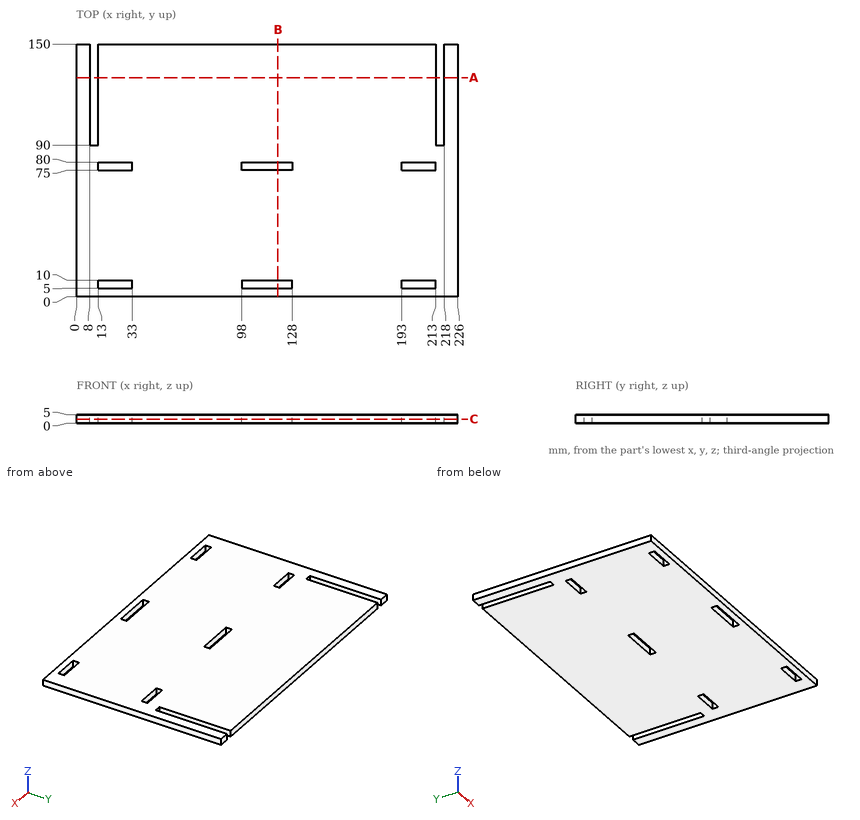
Study the drawing (mm; zero at the part's minimum x, y, z) and answer. Round coordinates to 2 decimals unless told otherwise and drop trailing zeros. Write each loop counter-clockwise with the first axis right and the second up, starting at its lowest first coordinate (ties: lowest second). Pieces come first, ordered by that corner, then holes.
Q1. Find section A-A on y = 130. Determine the outline of the cut face in (x, z), and give its area (3 significant figures).
Values:
outline: (0, 0) - (8, 0) - (8, 5) - (0, 5) - close; (13, 0) - (213, 0) - (213, 5) - (13, 5) - close; (218, 0) - (226, 0) - (226, 5) - (218, 5) - close
area: 1,080 mm2
Q2. Find section C-C on z = 2.55. State how many separate pieces and enclosed holes the cut face has, and give its area (3 significant figures).
Values:
separate pieces: 1
enclosed holes: 6
area: 32,600 mm2
Q3. Find section B-B on x = 119.5. Determine the outline of the cut face in (y, z), and give its area (3 significant figures).
Values:
outline: (0, 0) - (5, 0) - (5, 5) - (0, 5) - close; (10, 0) - (75, 0) - (75, 5) - (10, 5) - close; (80, 0) - (150, 0) - (150, 5) - (80, 5) - close
area: 700 mm2
Q4. A flat-ended cylindrical pin translates along its axis: P1, Ø2.5, axis at x = 9.5, z = 3.5, coming from the +Y side. Find the tip coordinate at first contact, or state that the pin passes through.
Values:
P1: stops at y = 90
Q5. Straight lines are drawn through the part: line 1 (X direction, y = 122, z = 4.5); line 2 (Y direction, x = 124.5, z = 2.5); line 3 (Y direction, x = 215, z = 4.4). For each, find the intervals that lie inside material, in ascending order.
Values:
line 1: x = 0 to 8, 13 to 213, 218 to 226
line 2: y = 0 to 5, 10 to 75, 80 to 150
line 3: y = 0 to 90
